```python
from build123d import *

# Parameters (mm, degrees)
SKETCH1_R           = 23.5
SKETCH1_R_2         = 15
BOSS_EXTRUDE1_DEPTH = 10
SKETCH2_R           = 30
SKETCH2_R_2         = 15
BOSS_EXTRUDE2_DEPTH = 10
CHAMFER1_SIZE       = 3
SKETCH3_R           = 5
BOSS_EXTRUDE3_DEPTH = 10


with BuildPart() as part:
    # Sketch1 → Boss-Extrude1 (new body)
    with BuildSketch(Plane.XY):
        Circle(SKETCH1_R)
        Circle(SKETCH1_R_2, mode=Mode.SUBTRACT)
    extrude(amount=-BOSS_EXTRUDE1_DEPTH)

    # Sketch2 → Boss-Extrude2 (add)
    with BuildSketch(Plane.XY):
        Circle(SKETCH2_R)
        Circle(SKETCH2_R_2, mode=Mode.SUBTRACT)
    extrude(amount=BOSS_EXTRUDE2_DEPTH)

    # Chamfer1
    chamfer1_edges = [part.edges().sort_by_distance(p)[0] for p in [
        (-23.5, 0, 0),
    ]]
    chamfer(chamfer1_edges, length=CHAMFER1_SIZE)

    # Sketch3 → Boss-Extrude3 (add)
    with BuildSketch(Plane.XY.offset(10)):
        with Locations((-22.5, 0)):
            Circle(SKETCH3_R)
        with Locations((22.5, 0)):
            Circle(SKETCH3_R)
    extrude(amount=BOSS_EXTRUDE3_DEPTH)


solid = part.part
```
Verification items for the finished model (mm, model axes). A direction names the side the tool comes from. Give positions to 0.01 mm unless a question says otherwise; leave off trailing zeros. Loops run counter-clockwise (first coordinate to the right, second up) from the corner with the lowest first, then second, coordinate; pieces in that order, holes last.
1. Set-up check for faces 4 (the cylindrical face through (17.505, 0.22, 14.93)), 5 (the cylindrical face through (22.4, 7.1, -6.5)), 6 (the flat face through (-0.3, -15.3, -10)): record each of +Z, -Z, +X, -X, +Y, -Y from which the full face is reachable in a straight line by a thin tool's end or side.
2. Mould release check, pull along X, two halves, no side actions. Record for faces 1 (the flat face through (-23, 0, 20)), 2 (the cylindrical face through (-27.495, 0.22, 14.93)), 3 (the conical face through (-3.08, 23.49, -2.81)): released by +X, released by -X, zero draft, split by the parting line, or undercut.
3. Section check B-B, the plane x = 0. Enter the section's corners in (y, z), then the cut area to 3 significant figures.
4. Section check D-D, the plane z = -1.75. Enter the section's corners in (x, y).
5. Thickness scan on line 1 (Y direction, x = 0, z = -4.5); line 2 (X direction, y = 10, z = 3.5); line 3 (Y direction, x = 11, z = -3.5). Record the ranges inside material, lowest first.
6. Section check C-C, the plane z = 18. Enter the section's corners in (x, y).
7. Go/stop test with flat-tipped pins: pin 1 Ø5 at (y, z) = (6, 1) entering from -X; pin 2 Ø24 at (x, y) = (0, 0) entering from +Z; pin 3 Ø2 at (y, z) = (-3.5, -7) entering from -X; pin 4 Ø4 at (y, z) = (11, 11) entering from -X. Record where each tip stops, or that it passes through.
8. Section check A-A, the plane y = 0. Enter the section's corners in (x, z), then the cut area to 3 significant figures.
Geometry says:
1. face 4: +Z
1. face 5: -Z
1. face 6: -Z, +X, -X, +Y, -Y
2. face 1: zero draft
2. face 2: undercut
2. face 3: split by the parting line
3. outline: (-30, 0) - (-26.5, 0) - (-23.5, -3) - (-23.5, -10) - (-15, -10) - (-15, 10) - (-30, 10) - close; (15, -10) - (23.5, -10) - (23.5, -3) - (26.5, 0) - (30, 0) - (30, 10) - (15, 10) - close
3. area: 479 mm2
4. outline: circle Ø49.5 at (0, 0); hole circle Ø30 at (0, 0)
5. line 1: y = -23.5 to -15, 15 to 23.5
5. line 2: x = -28.28 to -11.18, 11.18 to 28.28
5. line 3: y = -20.77 to -10.2, 10.2 to 20.77
6. outline: circle Ø10 at (-22.5, 0); circle Ø10 at (22.5, 0)
7. pin 1: stops at x = -29.8
7. pin 2: passes through
7. pin 3: stops at x = -23.37
7. pin 4: stops at x = -28.53
8. outline: (-30, 0) - (-26.5, 0) - (-23.5, -3) - (-23.5, -10) - (-15, -10) - (-15, 10) - (-17.5, 10) - (-17.5, 20) - (-27.5, 20) - (-27.5, 10) - (-30, 10) - close; (15, -10) - (23.5, -10) - (23.5, -3) - (26.5, 0) - (30, 0) - (30, 10) - (27.5, 10) - (27.5, 20) - (17.5, 20) - (17.5, 10) - (15, 10) - close
8. area: 679 mm2
